The listing builds one solid part. Answer for the finished solid, in the listing's coordinates (mm). Round coordinates to 2 decimals unless told otherwise and drop trailing zeros. Write each loop counter-clockwise with the first axis right and the second up, starting at its lowest first coordinate (ties: lowest second). Pieces come first, ordered by that corner, then holes.
Item 1: Find the intervals of material crossed by probe 1 along Y at (x, z) = (338, 25); probe 2 along X at (y, z) = (206, 45.5); probe 3 along X at (y, z) = (248, 31), in increasing order.
Item 2: For a pull along Z with two mould halves and no side action, classify faces 1 (the face through (400, -51, 76.2)), 2 (the face through (143, -6, 101.6)), 3 (the face through (143, -6, 0)) as +Z half, -Z half, draft (parallel to the pull), parting line (faces both ways), or undercut.
Item 3: Find section A-A on x = 336. Give the vertices of the cut face in (y, z).
Item 4: Find section C-C on z = 7.5. Give the vertices of the cut face in (x, y), then the cut area to 3 significant figures.
Item 5: Find section D-D on x = 408.5. Give the vertices of the cut face in (y, z), then the cut area to 3 significant figures.
Item 6: Each of these flat-tipped pins is pushed along its axis until it touches: pin 1 (6 mm diameter, centred on x = 211.5, z = 43, fed in from -Y); pin 2 (8 mm diameter, centred on x = 42.5, z = 87, fed in from +Y); pin 3 (12 mm diameter, centred on x = 420.5, z = 31, fed in from +Y). Where does it stop, or does it pass through?
Item 7: Find section B-B on y = -37.5. Give the vertices of the cut face in (x, z), then the cut area to 3 significant figures.
```python
from build123d import *

# Parameters (mm, degrees)
F1_DEPTH = 101.6
F3_DEPTH = 152.4
F4_W     = 143.211212
F4_H     = 118.549919
F5_DEPTH = 25.4


with BuildPart() as f1:
    # F0 (on Top) → F1 (new body)
    with BuildSketch(Plane.XY):
        with BuildLine():
            ThreePointArc((471.423321, -25.710636), (139.580084, 2.415757), (0.027949, 304.8))
            Line((0.027949, 304.8), (-6.35, 304.8))
            ThreePointArc((-6.35, 304.8), (136.074708, -2.881746), (473.906585, -31.560616))
            Line((473.906585, -31.560616), (471.423321, -25.710636))
        make_face()
    extrude(amount=F1_DEPTH)

    # F2 (on face) → F3 (cut)
    with BuildSketch(Plane(origin=(390.198528, 165.635729, 0), x_dir=(-0.390744, 0.9205, 0), z_dir=(0.9205, 0.390744, 0))):
        Polygon((-139.049853, 76.2), (-316.849853, 76.2), (-316.849853, 25.4), (-214.227537, 25.4), (-139.049853, 25.4), align=None)
    extrude(amount=-F3_DEPTH, mode=Mode.SUBTRACT)

    # F4 (on face) → F5 (cut)
    with BuildSketch(Plane(origin=(0, 304.8, 0), x_dir=(-1, 0, 0), z_dir=(0, 1, 0))):
        with Locations((-15.944215, 54.147762)):
            Rectangle(F4_W, F4_H)
    extrude(amount=-F5_DEPTH, mode=Mode.SUBTRACT)


solid = f1.part
```
Check values:
1. probe 1: y = -63.83 to -57.48
1. probe 2: x = -0.97 to 5.51
1. probe 3: x = -6.83 to -0.46
2. face 1: undercut
2. face 2: +Z half
2. face 3: -Z half
3. outline: (-63.88, 0) - (-57.52, 0) - (-57.52, 25.4) - (-63.88, 25.4) - close; (-63.88, 76.2) - (-57.52, 76.2) - (-57.52, 101.6) - (-63.88, 101.6) - close
4. outline: (-7.75, 279.4) arc R337.47 ccw to (473.91, -31.56) - (471.42, -25.71) arc R331.12 cw to (-1.4, 279.4) - close
4. area: 4,310 mm2
5. outline: (-54.6, 0) - (-48.07, 0) - (-48.07, 25.4) - (-54.6, 25.4) - close; (-54.6, 76.2) - (-48.07, 76.2) - (-48.07, 101.6) - (-54.6, 101.6) - close
5. area: 332 mm2
6. pin 1: stops at y = -43.67
6. pin 2: stops at y = 115.86
6. pin 3: stops at y = -44.26
7. outline: (198.74, 0) - (216.1, 0) - (216.1, 101.6) - (198.74, 101.6) - close; (443.24, 0) - (460.61, 0) - (460.61, 25.4) - (443.24, 25.4) - close; (443.24, 76.2) - (460.61, 76.2) - (460.61, 101.6) - (443.24, 101.6) - close
7. area: 2,650 mm2
